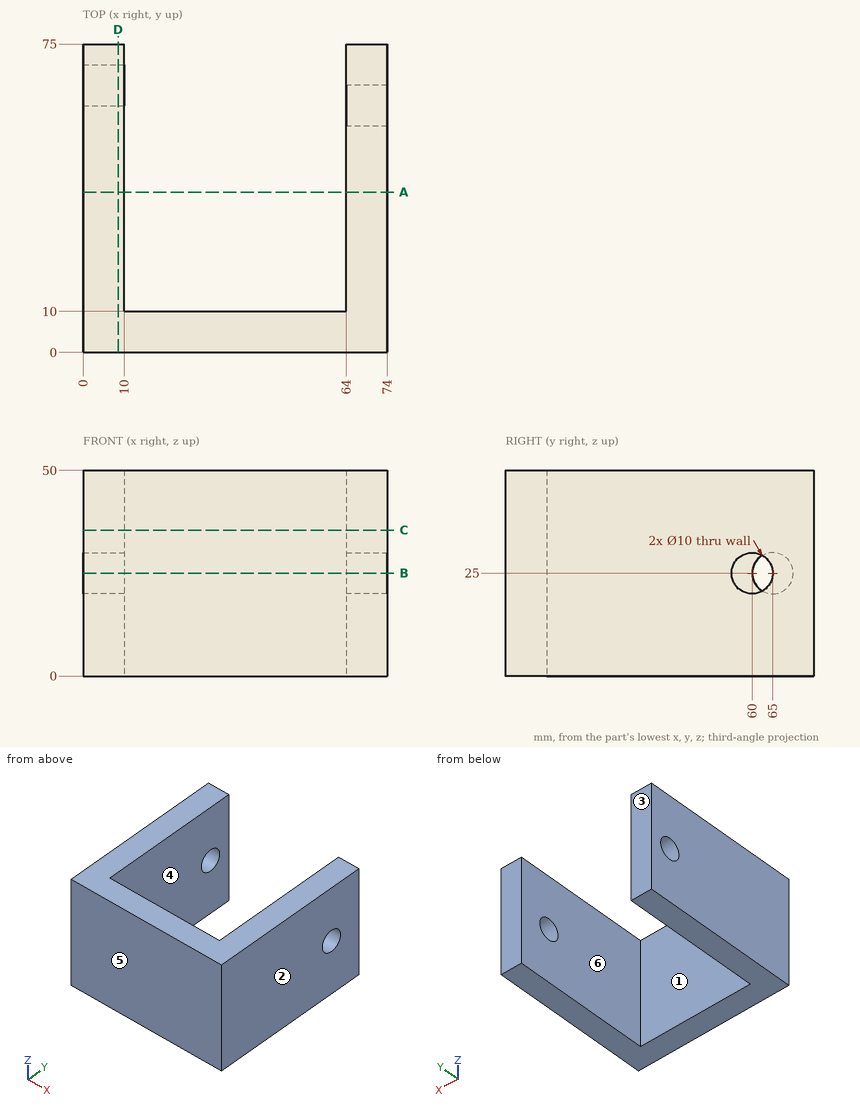
Source: three-view drawing plus pictorial views. Frame: mm from the lowest corner of the part. A direction names the side the tool comes from. Give positions to 0.01 mm unless a question says otherwise; leave off trailing zeros. Order: outer loops, then holes, each group sorted by start corner. A loop starts at its lowest first (then second) coordinate and runs counter-clockwise, first axis right, second up. Notation, with made-up numbers: (63, -29.5) -> (74, -29.5) arc R29 cw to (74, -2.5) -> close; hole circle Ø4 at (1, 57.25). An arc over 180 degrees is marked (long way). Write each question's results on one line, items separated by ' | '. Start each with the question number.
Item 1: Mould query, pull axis X, two halves, no side actions, for the marked faces 1, 2, 3 and 4. Classes: pulls with the +X half, pulls with the -X half, needs draft (parallel to the pull), parting line crosses it, or undercut.
Item 2: Cut plane C-C on z = 35.5. Return the cut outline in (x, y).
Item 3: Set-up query: the marked faces 5 and 6. Return all of +Z, -Z, +X, -X, +Y, -Y with unobstructed straight access to the full face (end or side cutting, diameter ignored); none if empty.
Item 4: Cut plane B-B on z = 25. Return the cut outline in (x, y).
Item 5: Cut plane D-D on x = 8.5. Return the cut outline in (y, z), then the cut area to 3 significant figures.
Item 6: Line query: line 1 (Y direction, x = 71.25, z = 25); line 2 (X direction, y = 59, z = 5); line 3 (Y direction, x = 5, z = 25). Output: solid intervals per line, ascending.
Item 7: Cut plane A-A on y = 39. Return the cut outline in (x, z), then the cut area to 3 significant figures.
Item 8: Contact query for a flat-ended pin moving along its axis: P1, Ø4, axis at x = 19, z = 28.5, coming from the +Y side. Output: stop coordinate, or through.
Established:
1) face 1: undercut | face 2: pulls with the +X half | face 3: needs draft | face 4: undercut
2) outline: (0, 0) -> (74, 0) -> (74, 75) -> (64, 75) -> (64, 10) -> (10, 10) -> (10, 75) -> (0, 75) -> close
3) face 5: +Z, -Z, +X, -X, -Y | face 6: +Z, -Z, +Y
4) outline: (0, 0) -> (74, 0) -> (74, 55) -> (64, 55) -> (64, 10) -> (10, 10) -> (10, 60) -> (0, 60) -> close; (0, 70) -> (10, 70) -> (10, 75) -> (0, 75) -> close; (64, 65) -> (74, 65) -> (74, 75) -> (64, 75) -> close
5) outline: (0, 0) -> (75, 0) -> (75, 50) -> (0, 50) -> close; hole circle Ø10 at (65, 25) | area: 3,670 mm^2
6) line 1: 0 to 55, 65 to 75 | line 2: 0 to 10, 64 to 74 | line 3: 0 to 60, 70 to 75
7) outline: (0, 0) -> (10, 0) -> (10, 50) -> (0, 50) -> close; (64, 0) -> (74, 0) -> (74, 50) -> (64, 50) -> close | area: 1,000 mm^2
8) P1: y = 10
